from build123d import *

# Parameters (mm, degrees)
SKETCH1_R           = 5.75
BOSS_EXTRUDE1_DEPTH = 3
BOSS_EXTRUDE2_DEPTH = 0.15
CIRPATTERN1_COUNT   = 2
SKETCH4_R           = 2.5
CUT_EXTRUDE1_DEPTH  = 7.0000001
FILLET1_R           = 0.5
CHAMFER1_SIZE       = 1


with BuildPart() as part:
    # Sketch1 → Boss-Extrude1 (new body, symmetric)
    with BuildSketch(Plane(origin=(0, 0, 0), x_dir=(1, 0, 0), z_dir=(0, 1, 0))):
        Circle(SKETCH1_R)
    extrude(amount=BOSS_EXTRUDE1_DEPTH, both=True)

    # Sketch3 → Boss-Extrude2 (add, symmetric)
    with BuildSketch(Plane(origin=(0, 0, 0), x_dir=(0.974370065, -0.224951054, 0), z_dir=(-0.224951054, -0.974370065, 0))):
        with BuildLine():
            Line((-7.260028368, 5.954486728), (-4.178380211, 2.872838571))
            add(Edge.make_bspline(
                [(0.674853163, 5.75), (-2.561446771, 5.75), (-4.178380211, 2.872838571)],
                knots=[0, 0, 0, 1.04763155, 1.04763155, 1.04763155], degree=2, weights=[1, 0.865916884, 1]))
            add(Edge.make_bspline(
                [(5.528086537, 2.872838571), (3.911153097, 5.75), (0.674853163, 5.75)],
                knots=[5.235553758, 5.235553758, 5.235553758, 6.283185307, 6.283185307, 6.283185307], degree=2, weights=[1, 0.865916884, 1]))
            add(Edge.make_bspline(
                [(5.528086537, 2.872838571), (5.499674649, 33.834937196), (3.406999963, 56.967753658), (3.396685559, 58.53294855)],
                knots=[0, 0, 0, 0, 0.918193758, 0.918193758, 0.918193758, 0.918193758], degree=3))
            ThreePointArc((3.396685559, 58.53294855), (1.920659701, 62.047163849), (-1.603205879, 63.5))
            Line((-1.603205879, 63.5), (-4.260028368, 63.5))
            ThreePointArc((-4.260028368, 63.5), (-6.381348711, 62.621320344), (-7.260028368, 60.5))
            Line((-7.260028368, 60.5), (-7.260028368, 5.954486728))
        make_face()
    boss_extrude2 = extrude(amount=BOSS_EXTRUDE2_DEPTH, both=True)

    # CirPattern1: Boss-Extrude2 ×2 about axis
    cirpattern1_axis = Axis((0, 3, 0), (0, -1, 0))
    for i in range(1, CIRPATTERN1_COUNT):
        add(boss_extrude2.rotate(cirpattern1_axis, i * 360 / CIRPATTERN1_COUNT))

    # Sketch4 → Cut-Extrude1 (cut, through all)
    with BuildSketch(Plane.XZ.offset(3)):
        Circle(SKETCH4_R)
    extrude(amount=-CUT_EXTRUDE1_DEPTH, mode=Mode.SUBTRACT)

    # Fillet1
    fillet1_edges = [part.edges().sort_by_distance(p)[0] for p in [
        (-5.75, -3, 0),
        (-5.75, 3, 0),
    ]]
    fillet(fillet1_edges, radius=FILLET1_R)

    # Chamfer1
    chamfer1_edges = [part.edges().sort_by_distance(p)[0] for p in [
        (-2.5, 3, 0),
        (-2.5, -3, 0),
    ]]
    chamfer(chamfer1_edges, length=CHAMFER1_SIZE)


solid = part.part
Verification items for the finished model (mm, model axes). Give positions to 0.01 mm unless a question says otherwise; leave off trailing zeros. Order: outer loops, then holes, each group sorted by start corner. A loop starts at its lowest first (then second) coordinate and runs counter-clockwise, first axis right, second up. Notation, with made-up numbers: (-38.75, 2) -> (14.25, 2) arc R31 ccw to (14.25, 41) -> close; hole circle Ø2 at (37, 86.5). An arc over 180 degrees is marked (long way). Answer as CSV lines item,"result".
Q1. Scan lines: probe 1 along Z at (x, y) = (0, 1.05); probe 2 along Y at (x, z) = (-4, -24); probe 3 along Z at (x, y) = (0, -0.05). Record each from-to range of solid material in increasing order.
Solutions:
probe 1,"z = -5.75 to -2.5, 2.5 to 5.75"
probe 2,"y = -1.08 to -0.77"
probe 3,"z = -63.23 to -2.5, 2.5 to 63.23"
Q2. Sectioned sample at A-A on z = 0. Record the cut outline in (x, y).
Solutions:
outline,"(-5.75, -2.5) arc R0.5 ccw to (-5.25, -3) -> (-3.5, -3) -> (-2.5, -2) -> (-2.5, 2) -> (-3.5, 3) -> (-5.25, 3) arc R0.5 ccw to (-5.75, 2.5) -> close; (2.5, -2) -> (3.5, -3) -> (5.25, -3) arc R0.5 ccw to (5.75, -2.5) -> (5.75, 2.5) arc R0.5 ccw to (5.25, 3) -> (3.5, 3) -> (2.5, 2) -> close"
Q3. Depth check by flat-ended pin: pin 1 (3 mm diameter, centred on x = 4.5, z = -17.5, fed in from +Y); pin 2 (4 mm diameter, centred on x = 5, z = -37.5, fed in from +Y); pin 3 (1.5 mm diameter, centred on x = -1.5, y = -1.5, fed in from +Z). Enter the tip coordinate at first touch or a pass-through.
Solutions:
pin 1,"stops at y = 1.54"
pin 2,"stops at y = 1.77"
pin 3,"stops at z = 5.7"
Q4. Release check for a two-part mould opening along X. For faces 1 (the flat face through (0, -3, -4)), 2 (the cylindrical face through (-0.54, -0.03, -2.44)) record: +X half, -X half, draft (parallel to the pull), parting line (faces both ways), or undercut.
Solutions:
face 1,"draft"
face 2,"undercut"
